Build history of the part. All positions in model axes, mm. A direction names the side the tool comes from. Round coordinates to 2 decimals unless told otherwise and drop trailing zeros. Write each loop counter-clockwise with the first axis right and the second up, starting at its lowest first coordinate (ties: lowest second). Pieces come first, ordered by that corner, then holes. Notation, with made-up numbers: M 55,-34 L 96,-34 A17 ccw 96,-21 Z; hole C -3.5,70 d5. An arc over 180 degrees is marked long. Write item = value, one per line. Start each with the question number.
Q1. Drop flat-ended pins along their axis: P1, Ø1.6, axis at x = 28, y = 5.5, coming from the +Z side; P2, Ø1.6, axis at x = 27, y = -4, coming from the +Z side. Give the stop position or say it passes through.
Q2. Band-saw the part on C-C on y = -2. Write the cut outline in (x, z), plus the area to 3 significant figures.
Q3. Band-saw the part on B-B on z = 0.55. Write the cut outline in (x, y).
Q4. Band-saw the part on D-D on y = 2. Write the cut outline in (x, z), plus the area to 3 significant figures.
Q5. Tool access for faces 1 (the flat face through (0, 0, 0)), 2 (the flat face through (-29, -2, 2)), 3 (the cylindrical face through (-28.55, -1.95, 2.25)), 4 (the cylindrical face through (-21.35, -6.56, 2.42)), 5 (the flat face through (30, 4.5, 3)): list every direction of +Z, -Z, +X, -X, +Y, -Y with a clear straight run to the whole face (end or side of a thin tool).
Q6. Band-saw the part on A-A on x = -27.45. Write the cut outline in (y, z).
Q7. Probe L1, parallel to Y at x = -27.45, z = 2.15; L2, parallel to X at y = 5.5, z = 1.7; L3, parallel to Y at x = -21, z = 0.65. List the from-to ranges inside material, lowest first.
```python
from build123d import *

# Parameters (mm, degrees)
SKETCH1_W           = 61.5
SKETCH1_H           = 16
BOSS_EXTRUDE1_DEPTH = 3.5
SKETCH5_W           = 60
SKETCH5_H           = 9
CUT_EXTRUDE3_DEPTH  = 1
SKETCH6_R           = 1.1
CUT_EXTRUDE4_DEPTH  = 32.871813566
SKETCH7_R           = 1.6
CUT_EXTRUDE5_DEPTH  = 2.2
SKETCH8_R           = 1.1
CUT_EXTRUDE6_DEPTH  = 32.871813566
SKETCH11_R          = 1.95
CUT_EXTRUDE10_DEPTH = 2


with BuildPart() as part:
    # Sketch1 → Boss-Extrude1 (new body)
    with BuildSketch(Plane.XY):
        Rectangle(SKETCH1_W, SKETCH1_H)
    extrude(amount=BOSS_EXTRUDE1_DEPTH)

    # Sketch5 → Cut-Extrude3 (cut)
    with BuildSketch(Plane.XY.offset(3.5)):
        with Locations((0.75, 0)):
            Rectangle(SKETCH5_W, SKETCH5_H)
    extrude(amount=-CUT_EXTRUDE3_DEPTH, mode=Mode.SUBTRACT)

    # Sketch6 → Cut-Extrude4 (cut, through all)
    with BuildSketch(Plane.XY.offset(2.5)):
        with Locations((-27.45, 2)):
            Circle(SKETCH6_R)
        with Locations((-27.45, -2)):
            Circle(SKETCH6_R)
        with Locations((23.05, 2)):
            Circle(SKETCH6_R)
    extrude(amount=-CUT_EXTRUDE4_DEPTH, mode=Mode.SUBTRACT)

    # Sketch7 → Cut-Extrude5 (cut)
    with BuildSketch(Plane.XY.offset(3.5)):
        with Locations((-21, 5)):
            Circle(SKETCH7_R)
        with Locations((-21, -5)):
            Circle(SKETCH7_R)
        with Locations((27.5, 5)):
            Circle(SKETCH7_R)
        with Locations((27.5, -5)):
            Circle(SKETCH7_R)
    extrude(amount=-CUT_EXTRUDE5_DEPTH, mode=Mode.SUBTRACT)

    # Sketch8 → Cut-Extrude6 (cut, through all)
    with BuildSketch(Plane.XY.offset(2.5)):
        with Locations((-21, 5)):
            Circle(SKETCH8_R)
        with Locations((-21, -5)):
            Circle(SKETCH8_R)
        with Locations((27.5, 5)):
            Circle(SKETCH8_R)
        with Locations((27.5, -5)):
            Circle(SKETCH8_R)
    extrude(amount=-CUT_EXTRUDE6_DEPTH, mode=Mode.SUBTRACT)

    # Sketch11 → Cut-Extrude10 (cut)
    with BuildSketch(Plane(origin=(0, 0, 0), x_dir=(-1, 0, 0), z_dir=(0, 0, -1))):
        with Locations((-23.05, 2)):
            Circle(SKETCH11_R)
        with Locations((27.45, -2)):
            Circle(SKETCH11_R)
        with Locations((27.45, 2)):
            Circle(SKETCH11_R)
    extrude(amount=-CUT_EXTRUDE10_DEPTH, mode=Mode.SUBTRACT)


solid = part.part
```
Conclusion:
q1.P1 = 1.3
q1.P2 = 2.5
q2.outline = M -30.75,0 L -29.4,0 L -29.4,2 L -28.55,2 L -28.55,2.5 L -29.25,2.5 L -29.25,3.5 L -30.75,3.5 Z; M -26.35,2 L -25.5,2 L -25.5,0 L 30.75,0 L 30.75,2.5 L -26.35,2.5 Z
q2.area = 146 mm^2
q3.outline = M -30.75,-8 L 30.75,-8 L 30.75,8 L -30.75,8 Z; hole C -27.45,-2 d3.9; hole C -27.45,2 d3.9; hole C -21,-5 d2.2; hole C -21,5 d2.2; hole C 23.05,2 d3.9; hole C 27.5,-5 d2.2; hole C 27.5,5 d2.2
q4.outline = M -30.75,0 L -29.4,0 L -29.4,2 L -28.55,2 L -28.55,2.5 L -29.25,2.5 L -29.25,3.5 L -30.75,3.5 Z; M -26.35,2 L -25.5,2 L -25.5,0 L 21.1,0 L 21.1,2 L 21.95,2 L 21.95,2.5 L -26.35,2.5 Z; M 24.15,2 L 25,2 L 25,0 L 30.75,0 L 30.75,2.5 L 24.15,2.5 Z
q4.area = 137 mm^2
q5.face_1 = -Z, +X, -X, +Y, -Y
q5.face_2 = -Z
q5.face_3 = +Z, -Z
q5.face_4 = +Z
q5.face_5 = +Z, +X
q6.outline = M -8,0 L -3.95,0 L -3.95,2 L -3.1,2 L -3.1,2.5 L -4.5,2.5 L -4.5,3.5 L -8,3.5 Z; M -0.9,2 L -0.05,2 L -0.05,0 L 0.05,0 L 0.05,2 L 0.9,2 L 0.9,2.5 L -0.9,2.5 Z; M 3.1,2 L 3.95,2 L 3.95,0 L 8,0 L 8,3.5 L 4.5,3.5 L 4.5,2.5 L 3.1,2.5 Z
q7.L1 = -8 to -3.1, -0.9 to 0.9, 3.1 to 8
q7.L2 = -30.75 to -22.52, -19.48 to 25.98, 29.02 to 30.75
q7.L3 = -8 to -6.1, -3.9 to 3.9, 6.1 to 8
